Model file for the job. Use its own axes, mm. A direction names the side the tool comes from. Round coordinates to 2 decimals unless told otherwise and drop trailing zeros. Loops run counter-clockwise (first coordinate to the right, second up) from the corner with the lowest first, then second, coordinate; pieces in that order, holes last. Notation, with made-up numbers: M -17,-4 L -6,-4 A26 cw -6,19 Z; hole C -20.5,8 d4. An arc over 180 degrees is marked long. Use a Markdown table: item, result. Add a question column.
Item 1: Pin check, flat tips, straight feed: P1, Ø4, axis at x = 16.5, z = 2.5, coming from the +Y side; P2, Ø6, axis at y = -6.5, z = 6.5, coming from the -X side; P3, Ø6.5, axis at x = 10.5, z = 4, coming from the +Y side. Stop position of each tip, or through.
Item 2: Saw through at D-D on z = 1.75. Write the cut outline in (x, y).
Item 3: Saw through at B-B on x = 5.25. Write the cut outline in (y, z), then the cut area to 3 significant figures.
Item 4: Saw through at A-A on y = -21. Write the cut outline in (x, z).
Item 5: Wall check: L1, parallel to Y at x = 20.2, z = 6.5; L2, parallel to Z at x = 0.95, y = -6.5; L3, parallel to X at y = -13, z = 8. Give the ranges that are in metal, low to high. Write a range as from..to.
Item 6: Two-plate mould, pull along Z, no slides. Class faces 1 (the cylindrical face through (18.972, -1.955, 1.854)), 2 (the cylindrical face through (10.4, -20, 6.4)), 3 (the flat face through (10, -25, 4)), 4 (the flat face through (10, -15, 6)): +Z half, -Z half, draft (parallel to the pull), parting line (faces both ways), or undercut.
Item 7: Saw through at C-C on y = -10. Write the cut outline in (x, z), then the cut area to 3 significant figures.
Item 8: Tool access for faces 5 (the cylindrical face through (12.408, -31.042, 7.101)), 6 (the cylindrical face through (10.353, -27.797, 4.363)), 7 (the flat face through (3, -9.3, 6.4)): list every direction of +Z, -Z, +X, -X, +Y, -Y with a clear straight run to the whole face (end or side of a thin tool).
```python
from build123d import *

# Parameters (mm, degrees)
BOSS_EXTRUDE1_DEPTH     = 13
CUT_EXTRUDE1_DEPTH      = 43.023802779
CUT_EXTRUDE2_DEPTH      = 43.023802779
CUT_EXTRUDE2_DEPTH_BACK = 43.023802779
SKETCH5_R               = 2.5
FILLET1_R               = 6.5
SKETCH6_R               = 2
CUT_EXTRUDE3_DEPTH      = 8


with BuildPart() as part:
    # Sketch2 → Boss-Extrude1 (new body)
    with BuildSketch(Plane.XY):
        Polygon((0, 0), (0, -34), (21, -34), (21, 0), (17, 0), (17, -15), (3, -15), (3, 0), align=None)
    extrude(amount=BOSS_EXTRUDE1_DEPTH)

    # Sketch4 → Cut-Extrude1 (cut, through all)
    with BuildSketch(Plane.ZY):
        with BuildLine():
            Line((4, -26.5), (4, -22.5))
            ThreePointArc((4, -22.5), (6.5, -20), (9, -22.5))
            Line((9, -22.5), (9, -26.5))
            ThreePointArc((9, -26.5), (6.5, -29), (4, -26.5))
        make_face()
    extrude(amount=-CUT_EXTRUDE1_DEPTH, mode=Mode.SUBTRACT)

    # Sketch5 → Cut-Extrude2 (cut, two sides: drawn at the far end of the back side and taken through both)
    with BuildSketch(Plane(origin=(21, 0, 0), x_dir=(0, 0, -1), z_dir=(1, 0, 0)).offset(-CUT_EXTRUDE2_DEPTH_BACK)):
        with Locations(Location((-6.5, -6.5, 0), (0, 0, 90))):
            Circle(SKETCH5_R)
    extrude(amount=CUT_EXTRUDE2_DEPTH + CUT_EXTRUDE2_DEPTH_BACK, mode=Mode.SUBTRACT)

    # Fillet1
    fillet1_edges = [part.edges().sort_by_distance(p)[0] for p in [
        (19, 0, 13),
        (1.5, 0, 13),
        (1.5, 0, 0),
        (19, 0, 0),
    ]]
    fillet(fillet1_edges, radius=FILLET1_R - 0.0001)  # a hair under: the kernel refuses the full size

    # Sketch6 → Cut-Extrude3 (cut)
    with BuildSketch(Plane.XZ.offset(34)):
        with Locations((10.5, 6.5)):
            Circle(SKETCH6_R)
    extrude(amount=-CUT_EXTRUDE3_DEPTH, mode=Mode.SUBTRACT)


solid = part.part
```
Entries:
| question | item | result |
|---|---|---|
| 1 | P1 | y = -0.34 |
| 1 | P2 | x = 0 |
| 1 | P3 | y = -15 |
| 2 | outline | M 0,-34 L 21,-34 L 21,-2.06 L 17,-2.06 L 17,-15 L 3,-15 L 3,-2.06 L 0,-2.06 Z |
| 3 | outline | M -34,0 L -15,0 L -15,13 L -34,13 Z; hole M -26.5,4 L -22.5,4 A2.5 ccw -22.5,9 L -26.5,9 A2.5 ccw Z |
| 3 | area | 207 mm2 |
| 4 | outline | M 0,0 L 21,0 L 21,4.5 L 0,4.5 Z; M 0,8.5 L 21,8.5 L 21,13 L 0,13 Z |
| 5 | L1 | -34..-29, -20..-9, -4..0 |
| 5 | L2 | 0..4, 9..13 |
| 5 | L3 | 0..3, 17..21 |
| 6 | face 1 | -Z half |
| 6 | face 2 | undercut |
| 6 | face 3 | undercut |
| 6 | face 4 | draft |
| 7 | outline | M 0,0 L 3,0 L 3,13 L 0,13 Z; M 17,0 L 21,0 L 21,13 L 17,13 Z |
| 7 | area | 91.0 mm2 |
| 8 | face 5 | -Y |
| 8 | face 6 | +X, -X |
| 8 | face 7 | +Z, -Z, +Y |
